Design review of the part built by this model. Coordinates are the model's own, in mm. A direction names the side the tool comes from. Coordinates: 2 decimals unless noted, no trailing zeros. Loops run counter-clockwise (first coordinate to the right, second up) from the corner with the lowest first, then second, coordinate; pieces in that order, holes last. Notation, with made-up numbers: (68.25, -32.5) - (94.25, -32.5) arc R21 ccw to (94.25, -10.5) - close; hole circle Ø8 at (34, 83). An arc over 180 degrees is marked (long way). Answer in a Markdown table with one row per item. Add a question column.
(1) The part is to be moulded in two halves that separate along Y. For faces 1 (the face through (-50, 53.98, -25.12)), 2 (the face through (-23, 660.4, -50)), 3 (the face through (-9, 326, -50.8)), say which applies: released by +Y, released by -Y, zero draft, split by the parting line, or undercut.
(2) We need section A-A, the plane y = 115.2. Write out the cut boundary in (x, z).
(3) We need section C-C, the plane y = 461. Write out the cut boundary in (x, z), plus the area to 4 significant figures.
(4) To check wall thickness, follow L1, parallel to X at y = 227, z = -13.5. State the ranges of the line that lie inside material, in increasing order. Write a range as [from, to].
(5) For faces 4 (the face through (-0.783, 380.997, -25.679)), 5 (the face through (-1.588, 326, -9)), 6 (the face through (-27.26, 559.366, -0.783)), list the 3-axis set-ups (+Z, -Z, +X, -X, +Y, -Y) from which the entire face can be reached by the end or side of a thin tool; tool diameter is ignored.
(6) We need section B-B, the plane z = -25.4. Give the number of separate pieces and of enclosed holes in the cut face, plus the area to 3 significant figures.
(7) Clearance check with a flat-ended pin moving along its axis: pin 1 (1 mm diameter, centred on x = -42.5, y = 238.5, fed in from +Z). State where the tip first meets the part, or that it passes through.
Autodesk Inventor part; units mm, degrees
ref_plane "YZ Plane" through (0, 0, 0) normal (1, 0, 0) x (0, 1, 0)
ref_plane "XZ Plane" through (0, 0, 0) normal (0, 1, 0) x (-1, 0, 0)
ref_plane "XY Plane" through (0, 0, 0) normal (0, 0, 1) x (1, 0, 0)
sketch "Sketch1" plane through (0, 0, 0) normal (0, 1, 0) x (-1, 0, 0)
  line L0 (0, 0) -> (50.8, 0)
  line L1 (50.8, 0) -> (50.8, -50.8)
  line L2 (50.8, -50.8) -> (0, -50.8)
  line L3 (0, -50.8) -> (0, 0)
  line L4 (49.2125, -1.5875) -> (1.5875, -1.5875)
  line L5 (1.5875, -1.5875) -> (1.5875, -49.2125)
  line L6 (1.5875, -49.2125) -> (49.2125, -49.2125)
  line L7 (49.2125, -49.2125) -> (49.2125, -1.5875)
  dimension "d0" = 50.8
  dimension "d1" = 50.8
  dimension "d2" = 1.5875
  dimension "d3" = 1.5875
  dimension "d4" = 1.5875
  dimension "d5" = 1.5875
extrude "Extrusion1" add sketch "Sketch1" along normal blind 660.4
sketch "Sketch2" plane through (-50.8, 0, 0) normal (0, 0, 1) x (1, 0, 0)
  line L0 (1.5875, 0) -> (49.2125, 0)
  line L1 (25.4, 0) -> (25.4, 660.4)
  line L2 (49.2125, 660.4) -> (1.5875, 660.4)
  line L3 (25.4, 0) -> (25.4, 104.775)
  line L4 (25.4, 660.4) -> (25.4, 555.625)
  circle A0 centre (25.4, 330.2) radius 14.2875
  line L5 (25.4, 330.2) -> (25.4, 115.2)
  line L6 (25.4, 330.2) -> (25.4, 545.2)
  circle A1 centre (25.4, 115.2) radius 14.2875
  circle A2 centre (25.4, 545.2) radius 14.2875
  point P0 (50.8, 0)
  dimension "d8" = 104.775
  dimension "d9" = 104.775
  dimension "d47" = 215
  dimension "d48" = 215
extrude "Extrusion2" cut sketch "Sketch2" against normal blind 530.225
sketch "Sketch3" plane through (-50.8, 0, 0) normal (0, 0, 1) x (1, 0, 0)
  circle A0 centre (25.4, 330.2) radius 14.2875
  circle A1 centre (16.4338, 257.9624) radius 2.54
  line L0 (16.4338, 257.9624) -> (6.9088, 257.9624)
  line L1 (16.4338, 257.9624) -> (25.9588, 257.9624)
  circle A2 centre (6.9088, 257.9624) radius 2.54
  circle A3 centre (25.9588, 257.9624) radius 2.54
  circle A4 centre (16.4338, 402.4376) radius 2.54
  circle A5 centre (6.9088, 402.4376) radius 2.54
  circle A6 centre (25.9588, 402.4376) radius 2.54
  line L2 (50.8, 0) -> (50.8, 660.4)
  line L3 (25.4, 330.2) -> (25.4, 344.4875)
  line L4 (16.4338, 399.8976) -> (16.4338, 402.4376)
  line L5 (25.4, 330.2) -> (25.4, 315.9125)
  line L6 (16.4338, 260.5024) -> (16.4338, 257.9624)
  dimension "d15" = 5.08
  dimension "d16" = 9.525
  dimension "d17" = 9.525
  dimension "d49" = 24.8412
  dimension "d50" = 9.525
  dimension "d51" = 9.525
  dimension "d52" = 72.2376
  dimension "d53" = 24.8412
  dimension "d54" = 72.2376
extrude "Extrusion3" cut sketch "Sketch3" against normal blind 101.6 contours L1 L6 A1 | A2 | A1 L0 L1 | A3 | L6 L0 A1 | A4 | A5 | A6
sketch "Sketch4" plane through (0, 0, 0) normal (1, 0, 0) x (0, 0, -1)
  circle A0 centre (25.4, 593.725) radius 12.7
  circle A1 centre (25.4, 517.525) radius 12.7
  line L0 (0, 660.4) -> (50.8, 660.4)
  line L1 (50.8, 0) -> (50.8, 660.4)
  line L2 (12.7, 593.725) -> (12.7, 517.525)
  line L3 (38.1, 517.525) -> (38.1, 593.725)
  point P0 (0, 0)
  dimension "d20" = 25.4
  dimension "d21" = 25.4
  dimension "d22" = 66.675
  dimension "d25" = 25.4
  dimension "d27" = 25.4
  dimension "d28" = 76.2
extrude "Extrusion4" cut sketch "Sketch4" against normal blind 127
sketch "Sketch5" plane through (0, 0, 0) normal (1, 0, 0) x (0, 0, -1)
  circle A0 centre (25.4, 66.675) radius 12.7
  circle A1 centre (25.4, 142.875) radius 12.7
  line L0 (50.8, 0) -> (0, 0)
  line L1 (0, 0) -> (0, 660.4)
  line L2 (50.8, 0) -> (50.8, 660.4)
  line L3 (12.7, 142.875) -> (12.7, 66.675)
  line L4 (38.1, 142.875) -> (38.1, 66.675)
  dimension "d31" = 25.4
  dimension "d32" = 25.4
  dimension "d33" = 66.675
  dimension "d34" = 25.4
  dimension "d35" = 25.4
  dimension "d36" = 76.2
extrude "Extrusion5" cut sketch "Sketch5" against normal blind 127
sketch "Sketch6" plane through (0, 0, 0) normal (1, 0, 0) x (0, 0, -1)
  circle A0 centre (25.4, 292.1) radius 12.7
  circle A1 centre (25.4, 368.3) radius 12.7
  line L0 (50.8, 0) -> (50.8, 660.4)
  line L1 (0, 0) -> (0, 660.4)
  line L2 (50.8, 0) -> (0, 0)
  line L3 (12.7, 368.3) -> (12.7, 292.1)
  line L4 (38.1, 368.3) -> (38.1, 292.1)
  dimension "d39" = 25.4
  dimension "d40" = 25.4
  dimension "d41" = 25.4
  dimension "d42" = 25.4
  dimension "d43" = 292.1
  dimension "d44" = 76.2
extrude "Extrusion6" cut sketch "Sketch6" against normal blind 127
properties part number "2x2x26" material "Aluminum 6061"
Responses:
| question | item | result |
|---|---|---|
| 1 | face 1 | undercut |
| 1 | face 2 | released by +Y |
| 1 | face 3 | zero draft |
| 2 | outline | (-50.8, -50.8) - (-39.69, -50.8) - (-39.69, -49.21) - (-49.21, -49.21) - (-49.21, -38.1) - (-50.8, -38.1) - close; (-50.8, -12.7) - (-49.21, -12.7) - (-49.21, -1.59) - (-39.69, -1.59) - (-39.69, 0) - (-50.8, 0) - close; (-11.11, -50.8) - (0, -50.8) - (0, -38.1) - (-1.59, -38.1) - (-1.59, -49.21) - (-11.11, -49.21) - close; (-11.11, -1.59) - (-1.59, -1.59) - (-1.59, -12.7) - (0, -12.7) - (0, 0) - (-11.11, 0) - close |
| 3 | outline | (-50.8, -50.8) - (0, -50.8) - (0, 0) - (-50.8, 0) - close; hole (-49.21, -49.21) - (-1.59, -49.21) - (-1.59, -1.59) - (-49.21, -1.59) - close |
| 3 | area | 312.5 mm2 |
| 4 | L1 | x = [-50.8, -49.21], [-1.59, 0] |
| 5 | face 4 | +X, -X |
| 5 | face 5 | +Y, -Y |
| 5 | face 6 | +Z, -Z |
| 6 | separate pieces | 8 |
| 6 | enclosed holes | 0 |
| 6 | area | 1,130 mm2 |
| 7 | pin 1 | stops at z = 0 |
